from build123d import *

# Parameters (mm, degrees)
SKETCH_1_R      = 1.75
SKETCH_1_R_2    = 2
SKETCH_1_R_3    = 1.5
EXTRUDE_1_DEPTH = 3


with BuildPart() as part:
    # 草图1 → 凸台-拉伸1 (new body)
    with BuildSketch(Plane(origin=(0, 0, 0), x_dir=(1, 0, 0), z_dir=(0, 1, 0))):
        with BuildLine():
            Line((-45, 50), (45, 50))
            ThreePointArc((45, 50), (48.535533906, 48.535533906), (50, 45))
            Line((50, 45), (50, -45))
            ThreePointArc((50, -45), (48.535533906, -48.535533906), (45, -50))
            Line((45, -50), (-45, -50))
            ThreePointArc((-45, -50), (-48.535533906, -48.535533906), (-50, -45))
            Line((-50, -45), (-50, 45))
            ThreePointArc((-50, 45), (-48.535533906, 48.535533906), (-45, 50))
        make_face()
        with Locations(Location((-45, 45, 0), (0, 0, 270))):
            Circle(SKETCH_1_R, mode=Mode.SUBTRACT)
        with Locations(Location((45, 45, 0), (0, 0, 270))):
            Circle(SKETCH_1_R, mode=Mode.SUBTRACT)
        with Locations(Location((-45, -45, 0), (0, 0, 270))):
            Circle(SKETCH_1_R, mode=Mode.SUBTRACT)
        with Locations(Location((45, -45, 0), (0, 0, 270))):
            Circle(SKETCH_1_R, mode=Mode.SUBTRACT)
        with Locations(Location((12, 10.5, 0), (0, 0, 270))):
            Circle(SKETCH_1_R, mode=Mode.SUBTRACT)
        with Locations(Location((42, 10.5, 0), (0, 0, 270))):
            Circle(SKETCH_1_R, mode=Mode.SUBTRACT)
        with Locations(Location((12, -13.5, 0), (0, 0, 270))):
            Circle(SKETCH_1_R, mode=Mode.SUBTRACT)
        with Locations(Location((42, -13.5, 0), (0, 0, 270))):
            Circle(SKETCH_1_R, mode=Mode.SUBTRACT)
        with Locations(Location((-42, 13.5, 0), (0, 0, 270))):
            Circle(SKETCH_1_R, mode=Mode.SUBTRACT)
        with Locations(Location((-12, 13.5, 0), (0, 0, 270))):
            Circle(SKETCH_1_R, mode=Mode.SUBTRACT)
        with Locations(Location((-42, -10.5, 0), (0, 0, 270))):
            Circle(SKETCH_1_R, mode=Mode.SUBTRACT)
        with Locations(Location((-12, -10.5, 0), (0, 0, 270))):
            Circle(SKETCH_1_R, mode=Mode.SUBTRACT)
        with Locations(Location((-14, -35.5, 0), (0, 0, 270))):
            Circle(SKETCH_1_R_2, mode=Mode.SUBTRACT)
        with Locations(Location((14, -35.5, 0), (0, 0, 270))):
            Circle(SKETCH_1_R_2, mode=Mode.SUBTRACT)
        with Locations(Location((-14, 35.5, 0), (0, 0, 270))):
            Circle(SKETCH_1_R_2, mode=Mode.SUBTRACT)
        with Locations(Location((14, 35.5, 0), (0, 0, 270))):
            Circle(SKETCH_1_R_2, mode=Mode.SUBTRACT)
        with Locations(Location((-39.5, 33.25, 0), (0, 0, 270))):
            Circle(SKETCH_1_R_3, mode=Mode.SUBTRACT)
        with Locations(Location((39.5, 33.25, 0), (0, 0, 270))):
            Circle(SKETCH_1_R_3, mode=Mode.SUBTRACT)
        with Locations(Location((-39.5, -33.25, 0), (0, 0, 270))):
            Circle(SKETCH_1_R_3, mode=Mode.SUBTRACT)
        with Locations(Location((39.5, -33.25, 0), (0, 0, 270))):
            Circle(SKETCH_1_R_3, mode=Mode.SUBTRACT)
    extrude(amount=EXTRUDE_1_DEPTH)


solid = part.part
Read the model definition and answer for the solid it produces. Units are mm, in the model's axes. Coordinates: 2 decimals unless noted, no trailing zeros. Write each loop counter-clockwise with the first axis right and the second up, starting at its lowest first coordinate (ties: lowest second). Pieces come first, ordered by that corner, then holes. Notation, with made-up numbers: M 75.25,10.5 L 88.25,10.5 A20 ccw 88.25,31.5 Z; hole C 25.5,64.5 d11. An arc over 180 degrees is marked long. Use a Markdown table: item, result.
Q1. The part is cut by section B-B, the plane y = 1.2. Give the number of separate pieces and of enclosed holes in the cut face, then the cut area to 3 significant figures.
Answer block:
| item | result |
|---|---|
| separate pieces | 1 |
| enclosed holes | 20 |
| area | 9,780 mm2 |
Q2. The part is cut by section A-A, the plane z = -13.5. Write down the section's boundary in (x, y).
Answer block:
| item | result |
|---|---|
| outline | M -50,0 L -43.75,0 L -43.75,3 L -50,3 Z; M -40.25,0 L -13.75,0 L -13.75,3 L -40.25,3 Z; M -10.25,0 L 50,0 L 50,3 L -10.25,3 Z |
Q3. Straight lines are drawn through the part: L1, parallel to X at y = 1.9, z = -45; L2, parallel to X at y = 1.1, z = 13.5; L3, parallel to Z at x = 44, y = 2.5. For each, find the intervals that lie inside material, in ascending order. Write a range as [from, to].
Answer block:
| item | result |
|---|---|
| L1 | x = [-50, -46.75], [-43.25, 43.25], [46.75, 50] |
| L2 | x = [-50, 10.25], [13.75, 40.25], [43.75, 50] |
| L3 | z = [-50, -46.44], [-43.56, 43.56], [46.44, 50] |
Q4. Determine the mould class of faces 1 (the face through (-40.41, 1.48, -34.44)), 2 (the face through (40.29, 1.48, -10.88)), 3 (the face through (1, 3, -1)), 4 (the face through (48, 1, -49)) for opening direction X: released by +X, released by -X, zero draft, split by the parting line, or undercut.
Answer block:
| item | result |
|---|---|
| face 1 | undercut |
| face 2 | undercut |
| face 3 | zero draft |
| face 4 | released by +X |
